Work out the finished part from the listing and answer in its coordinate system (mm). Face numbers are marked on the shaded views. A direction names the side the tool comes from. Give positions to 0.01 mm unless a question says otherwise; leave off trailing zeros. Order: outer loops, then holes, each group sorted by start corner. A loop starts at its lowest first (then second) coordinate and runs counter-clockwise, first axis right, second up.
```python
from build123d import *

# Parameters (mm, degrees)
BASE_FLANGE1_DEPTH                     = 30
F_3_0MM_TRANSITIONAL_DOWEL_HOLE1_D     = 3
F_3_0MM_TRANSITIONAL_DOWEL_HOLE1_DEPTH = 1.5
F_3_0MM_TRANSITIONAL_DOWEL_HOLE2_D     = 3
F_3_0MM_TRANSITIONAL_DOWEL_HOLE2_DEPTH = 1.5
F_3_0MM_PRESS_DOWEL_HOLE1_D            = 3
F_3_0MM_PRESS_DOWEL_HOLE1_DEPTH        = 6
F_3_0MM_PRESS_DOWEL_HOLE1_TIP          = 0.901290929


# Sheet-metal steps are written as plain solids
with BuildPart() as part:
    # Sketch1 → Base-Flange1 (new body)
    with BuildSketch(Plane(origin=(0, 0, 0), x_dir=(1, 0, 0), z_dir=(0, 1, 0))):
        with BuildLine():
            Line((0, 0), (17.7634, 0))
            ThreePointArc((17.7634, 0), (19.344915027, -0.655084973), (20, -2.2366))
            Line((20, -2.2366), (20, -41.7634))
            ThreePointArc((20, -41.7634), (19.344915027, -43.344915027), (17.7634, -44))
            Line((17.7634, -44), (-10, -44))
            Line((-10, -44), (-10, -42.5))
            Line((-10, -42.5), (17.7634, -42.5))
            ThreePointArc((17.7634, -42.5), (18.284254855, -42.284254855), (18.5, -41.7634))
            Line((18.5, -41.7634), (18.5, -2.2366))
            ThreePointArc((18.5, -2.2366), (18.284254855, -1.715745145), (17.7634, -1.5))
            Line((17.7634, -1.5), (0, -1.5))
            Line((0, -1.5), (0, 0))
        make_face()
    extrude(amount=BASE_FLANGE1_DEPTH)

    # Ø3.0mm Transitional Dowel Hole1
    with Locations(Plane(origin=(0, 0, 0), x_dir=(-1, 0, 0), z_dir=(0, 0, -1))):
        with Locations((-10, 25), (-10, 5)):
            Hole(F_3_0MM_TRANSITIONAL_DOWEL_HOLE1_D / 2, depth=F_3_0MM_TRANSITIONAL_DOWEL_HOLE1_DEPTH)

    # Ø3.0mm Transitional Dowel Hole2
    with Locations(Plane.XY.offset(44)):
        with Locations((5, 15)):
            Hole(F_3_0MM_TRANSITIONAL_DOWEL_HOLE2_D / 2, depth=F_3_0MM_TRANSITIONAL_DOWEL_HOLE2_DEPTH)

    # Ø3.0mm Press Dowel Hole1
    with Locations(Plane(origin=(146.531359221, 116.2862719, -6), x_dir=(0, -1, 0), z_dir=(0, 0, -1))):
        with Locations((220.525513363, 156.531359221), (102.525513363, 181.531359221), (102.525513363, 271.531359221), (89.19270005, 226.531359221), (210.525513363, 317.793651488), (230.525513363, 317.793651488), (252.525513363, 320.462332131), (232.525513363, 300.462332131), (252.525513363, 132.600386311), (232.525513363, 152.600386311), (111.286271896, 136.531359221), (91.286271896, 136.531359221), (41.525513363, 196.432813402), (13.525513363, 196.432813402), (41.525513363, 138.767959221), (13.525513363, 138.767959221), (41.525513363, 256.62990504), (13.525513363, 256.62990504), (41.525513363, 314.294759221), (13.525513363, 314.294759221)):
            Hole(F_3_0MM_PRESS_DOWEL_HOLE1_D / 2, depth=F_3_0MM_PRESS_DOWEL_HOLE1_DEPTH)
            with Locations((0, 0, -(F_3_0MM_PRESS_DOWEL_HOLE1_DEPTH + F_3_0MM_PRESS_DOWEL_HOLE1_TIP / 2))):  # 118° drill point
                Cone(0, F_3_0MM_PRESS_DOWEL_HOLE1_D / 2, F_3_0MM_PRESS_DOWEL_HOLE1_TIP, mode=Mode.SUBTRACT)


solid = part.part
```
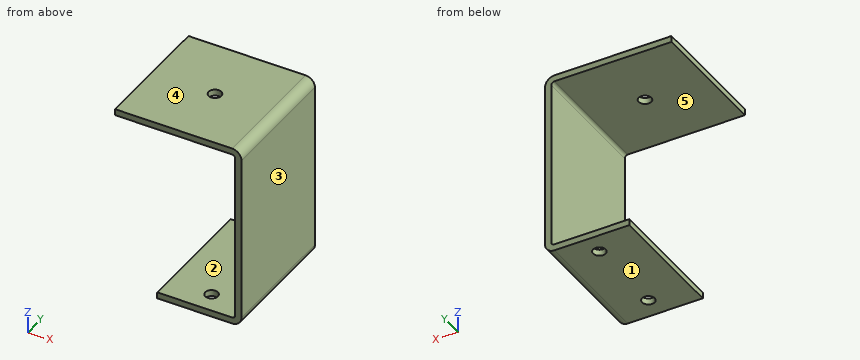
1. Straight lines are drawn through the part: probe 1 along Y at (x, z) = (10, 0.7); probe 2 along Z at (x, y) = (8.5, 7.5); probe 3 along Y at (x, z) = (5, 43). For each, find the intervals that lie inside material, in ascending order.
Findings below:
probe 1: y = 0 to 3.5, 6.5 to 23.5, 26.5 to 30
probe 2: z = 0 to 1.5, 42.5 to 44
probe 3: y = 0 to 13.5, 16.5 to 30
2. The part is cut by section C-C (x = 5). Write down the section's boundary in (y, z).
Findings below:
outline: (0, 0) - (30, 0) - (30, 1.5) - (0, 1.5) - close; (0, 42.5) - (13.5, 42.5) - (13.5, 44) - (0, 44) - close; (16.5, 42.5) - (30, 42.5) - (30, 44) - (16.5, 44) - close
3. The part is cut by section B-B (x = 15). Write down the section's boundary in (y, z), then the cut area to 3 significant figures.
Findings below:
outline: (0, 0) - (30, 0) - (30, 1.5) - (0, 1.5) - close; (0, 42.5) - (30, 42.5) - (30, 44) - (0, 44) - close
area: 90.0 mm2
4. The part is cut by section A-A (y = 15). Write down the section's boundary in (x, z), then the cut area to 3 significant figures.
Findings below:
outline: (-10, 42.5) - (3.5, 42.5) - (3.5, 44) - (-10, 44) - close; (0, 0) - (17.76, 0) arc R2.24 ccw to (20, 2.24) - (20, 41.76) arc R2.24 ccw to (17.76, 44) - (6.5, 44) - (6.5, 42.5) - (17.76, 42.5) arc R0.74 cw to (18.5, 41.76) - (18.5, 2.24) arc R0.74 cw to (17.76, 1.5) - (0, 1.5) - close
area: 130 mm2
5. Which of the six approach directions +Z, -Z, +X, -X, +Y, -Y give full straight-line access (tool end or side, diameter ignored) to the marked faces 4 and 5?
Findings below:
face 4: +Z, +X, -X, +Y, -Y
face 5: -X, +Y, -Y
6. The part is cut by section D-D (y = 21.75). Write down the section's boundary in (x, z).
Findings below:
outline: (-10, 42.5) - (17.76, 42.5) arc R0.74 cw to (18.5, 41.76) - (18.5, 2.24) arc R0.74 cw to (17.76, 1.5) - (0, 1.5) - (0, 0) - (17.76, 0) arc R2.24 ccw to (20, 2.24) - (20, 41.76) arc R2.24 ccw to (17.76, 44) - (-10, 44) - close
7. Given P1, Ø2, axis at y = 13, z = 28.5, coming from the -X side; P2, Ø1.6, axis at y = 15.5, z = 1, coming from the -X side; P3, Ø2.5, axis at x = 10, y = 5, coming from the -Z side, each flat-ended and moving along its own axis, determine where each tip first touches the part or whether it passes through.
Findings below:
P1: stops at x = 18.5
P2: stops at x = 0
P3: stops at z = 42.5
8. The mould has two halves that part along Z. Classify the marked faces 1, 2 and 3: pulls with the +Z half, pulls with the -Z half, needs draft (parallel to the pull), parting line crosses it, or undercut.
Findings below:
face 1: pulls with the -Z half
face 2: undercut
face 3: needs draft
